Model file for the job. Use its own axes, mm. A direction names the side the tool comes from. Round coordinates to 2 decimals unless told otherwise and drop trailing zeros. Order: outer loops, then holes, each group sorted by start corner. A loop starts at its lowest first (then second) coordinate and runs counter-clockwise, first axis right, second up. Notation, with made-up numbers: (73.25, 13.25) - (116.25, 13.25) arc R20 cw to (116.25, 46.25) - close; hole circle Ø1 at (84, 52.5). An arc over 180 degrees is marked (long way). Use one line per item in the form item = value.
from build123d import *

# Parameters (mm, degrees)
F0_W     = 35
F0_H     = 39.2
F1_DEPTH = 84
F3_DEPTH = 69
F5_D     = 5.5
F6_W     = 35
F6_H     = 10.8
F7_DEPTH = 84.001


with BuildPart() as f1:
    # F0 (on Front) → F1 (new body)
    with BuildSketch(Plane.XZ):
        Rectangle(F0_W, F0_H)
    extrude(amount=F1_DEPTH)

    # F2 (on face) → F3 (cut)
    with BuildSketch(Plane.XZ.offset(84)):
        Polygon((12.62, -3.3), (12.62, 3.3), (6.8694977982, 3.3), (6.8694977982, 8.8), (-6.8694977982, 8.8), (-6.8694977982, 3.3), (-12.62, 3.3), (-12.62, -3.3), align=None)
    extrude(amount=-F3_DEPTH, mode=Mode.SUBTRACT)

    # F5 (through all)
    with Locations(Plane(origin=(0, 0, 0), x_dir=(-1, 0, 0), z_dir=(0, 1, 0))):
        with Locations((0, 0.7)):
            Hole(F5_D / 2)

    # F6 (on face) → F7 (cut, through all)
    with BuildSketch(Plane.XZ.offset(84)):
        with Locations((0, 14.2)):
            Rectangle(F6_W, F6_H)
    extrude(amount=-F7_DEPTH, mode=Mode.SUBTRACT)


solid = f1.part
(1) Slice it at D-D on y = -43.5. Give the cut face in (x, z), then the cut area to 3 significant figures.
Report:
outline = (-17.5, -19.6) - (17.5, -19.6) - (17.5, 8.8) - (6.87, 8.8) - (6.87, 3.3) - (12.62, 3.3) - (12.62, -3.3) - (-12.62, -3.3) - (-12.62, 3.3) - (-6.87, 3.3) - (-6.87, 8.8) - (-17.5, 8.8) - close
area = 752 mm2
(2) Slice it at B-B on x = 0. Give the cut face in (y, z).
Report:
outline = (-84, -19.6) - (0, -19.6) - (0, -2.05) - (-15, -2.05) - (-15, -3.3) - (-84, -3.3) - close; (-15, 3.45) - (0, 3.45) - (0, 8.8) - (-15, 8.8) - close
(3) Slice it at A-A on z = 0.7. Give the cut face in (x, y).
Report:
outline = (-17.5, -84) - (-12.62, -84) - (-12.62, -15) - (-2.75, -15) - (-2.75, 0) - (-17.5, 0) - close; (2.75, -15) - (12.62, -15) - (12.62, -84) - (17.5, -84) - (17.5, 0) - (2.75, 0) - close
(4) Pin check, flat tip, straight feed: pin 1 (8 mm diameter, centred on x = -2, y = -45.5, fed in from +Z). Stop position of the tip, or through.
Report:
pin_1 = -3.3
(5) Tool access for faces 1 (the face through (0, -41, -19.6)), 2 (the face through (6.869, -50, 6)), 3 (the face through (-10, -50, 3.3)): list every direction of +Z, -Z, +X, -X, +Y, -Y with a clear straight run to the whole face (end or side of a thin tool).
Report:
face_1 = -Z, +X, -X, +Y, -Y
face_2 = +Z, -Y
face_3 = -Y
(6) Slice it at C-C on y = -7. Give the cut face in (x, z), then the cut area to 3 significant figures.
Report:
outline = (-17.5, -19.6) - (17.5, -19.6) - (17.5, 8.8) - (-17.5, 8.8) - close; hole circle Ø5.5 at (0, 0.7)
area = 970 mm2
(7) Pull direction Z, two halves, no side cores. Call faces 4 (the face through (17.5, -41, -6)), 5 (the face through (8, -43, 8.8)), 6 (the face through (0, -50, -3.3)): released by +Z, released by -Z, zero draft, split by the parting line, or undercut.
Report:
face_4 = zero draft
face_5 = released by +Z
face_6 = undercut
(8) Probe probe 1 along Z at (x, y) = (0, -10.25); probe 2 along X at (y, z) = (-75, 5.25); probe 3 along Z at (x, y) = (12.5, -78). List the from-to ranges inside material, lowest first. Write a range as [from, to].
Report:
probe_1 = [-19.6, -2.05], [3.45, 8.8]
probe_2 = [-17.5, -6.87], [6.87, 17.5]
probe_3 = [-19.6, -3.3], [3.3, 8.8]
